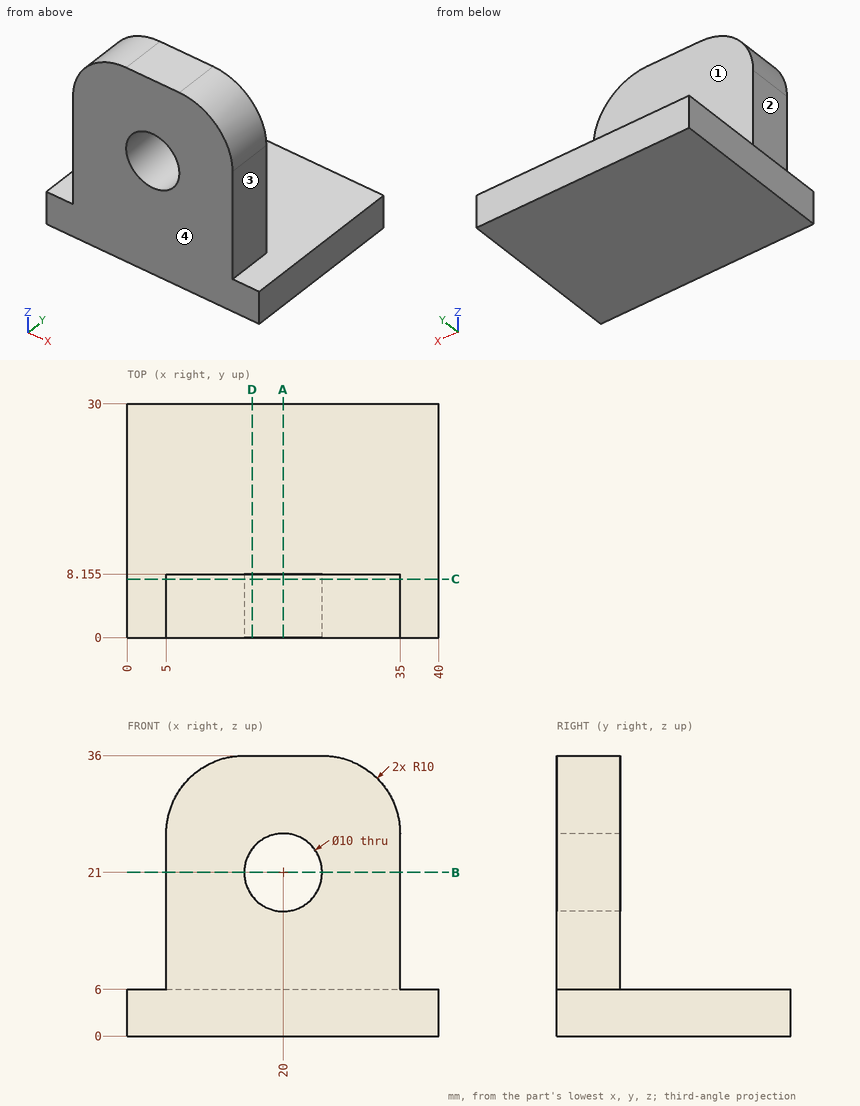
Design review of the part shown in the three views and the two pictorial views. Dimensions are in mm from the part's minimum x, y and z. A direction names the side the tool comes from. Coordinates: 2 decimals unless noted, no trailing zeros. Order: outer loops, then holes, each group sorted by start corner. A loop starts at its lowest first (then second) coordinate and runs counter-clockwise, first axis right, second up.
1) Take a section at A-A, the plane x = 20. Give the boundary of the cut face in (y, z) (1 decimal), and give its area (3 significant figures).
2) For the marked faces 1, 2, 3 and 4, list the 3-axis set-ups (+Z, -Z, +X, -X, +Y, -Y) from which the entire face can be reached by the end or side of a thin tool; tool diameter is ignored.
3) Take a section at D-D, the plane x = 16. Give the boundary of the cut face in (y, z) (1 decimal), and give its area (3 significant figures).
4) Clearance check with flat-ended pins moving along their axes: pin 1 (6 mm diameter, centred on x = 28.5, z = 19.5, fed in from +Y) (3 decimals); pin 2 (1 mm diameter, centred on x = 24.5, y = 9.5, fed in from +Z); pin 3 (4 mm diameter, centred on y = 3, z = 11, fed in from -X). State where each tip first meets the part, or that it passes through.
5) Take a section at C-C, the plane y = 7.5. Give the boundary of the cut face in (x, z), and give its area (3 significant figures).
6) Take a section at B-B, the plane z = 21. Give the boundary of the cut face in (x, y) (1 decimal).
7) Wall thickness on line 1 along Z through (x, y) = (20, 2.75); line 2 along Z through (x, y) = (16, 10); line 3 along X through (y, z) = (4.75, 11): over which ranges is each line inside the solid? List them lowest first.
Returned:
1. outline: (0, 0) - (30, 0) - (30, 6) - (8.2, 6) - (8.2, 16) - (0, 16) - close; (0, 26) - (8.2, 26) - (8.2, 36) - (0, 36) - close
1. area: 343 mm2
2. face 1: +Z, +X, -X, +Y
2. face 2: +Z, -X, +Y, -Y
2. face 3: +Z, +X, +Y, -Y
2. face 4: +Z, -Z, +X, -X, -Y
3. outline: (0, 0) - (30, 0) - (30, 6) - (8.2, 6) - (8.2, 18) - (0, 18) - close; (0, 24) - (8.2, 24) - (8.2, 36) - (0, 36) - close
3. area: 376 mm2
4. pin 1: stops at y = 8.155
4. pin 2: stops at z = 6
4. pin 3: stops at x = 5
5. outline: (0, 0) - (40, 0) - (40, 6) - (35, 6) - (35, 26) arc R10 ccw to (25, 36) - (15, 36) arc R10 ccw to (5, 26) - (5, 6) - (0, 6) - close; hole circle Ø10 at (20, 21)
5. area: 1,020 mm2
6. outline: (5, 0) - (15, 0) - (15, 8.2) - (5, 8.2) - close; (25, 0) - (35, 0) - (35, 8.2) - (25, 8.2) - close
7. line 1: z = 0 to 16, 26 to 36
7. line 2: z = 0 to 6
7. line 3: x = 5 to 35
